The figure shows three views and two pictorial views of one solid part (mm, origin at its lowest corner). Answer the questions. A direction names the side the tool comes from. Give positions to 0.01 mm unless a question says otherwise; leave off trailing zeros. Write each loop counter-clockwise with the first axis right and the second up, starting at its lowest first coordinate (ties: lowest second). Pieces come first, ordered by that corner, then holes. Notation, with made-up numbers: (82.25, -27) -> (89.25, -27) arc R23 ccw to (89.25, 8) -> close; hole circle Ø10 at (-34, 67). An arc over 180 degrees is marked (long way). Write item = value, one per line. Start each with the question number.
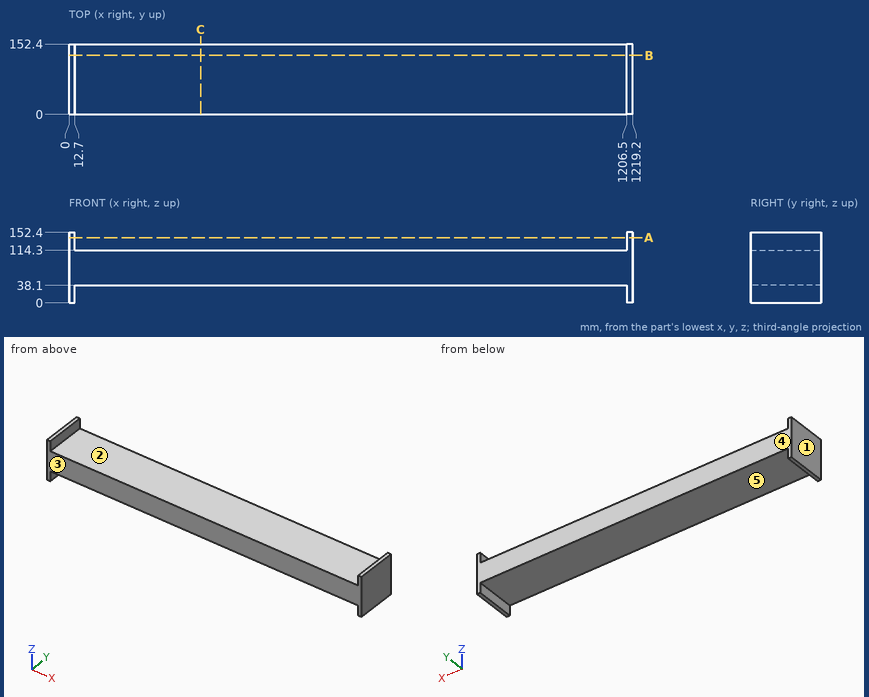
(1) For the marked faces 1 and 2, determine the directions among +Z, -Z, +X, -X, +Y, -Y from which every point of the face is accessible in a straight line to the end or side of a thin tool.
(2) This flat-tipped pin is pushed along its axis until it touches: pin 1 (4 mm diameter, centred on x = 228.5, y = 86, fed in from +Z). Where does it stop, or does it pass through?
(3) Find the intervals of material crossed by line 1 along X through (y, z) = (17.5, 134); line 2 along Z through (x, y) = (523.5, 63.5), in increasing order.
(4) A cutting plane is placed at C-C, the plane x = 285. Write down the section's boundary in (y, z).
(5) Determine the mould class of the marked faces 3, 4 and 5 for opening direction Y: pulls with the +Y half, pulls with the -Y half, needs draft (parallel to the pull), parting line crosses it, or undercut.
(6) A cutting plane is placed at B-B, the plane y = 128. Write down the section's boundary in (x, z), then the cut area to 3 significant figures.
(7) A cutting plane is placed at A-A, the plane z = 141. Write down the section's boundary in (x, y).
Results list:
q1.face_1 = +Z, -Z, -X, +Y, -Y
q1.face_2 = +Z, +Y, -Y
q2.pin_1 = 114.3
q3.line_1 = 0 to 12.7, 1206.5 to 1219.2
q3.line_2 = 38.1 to 114.3
q4.outline = (0, 38.1) -> (152.4, 38.1) -> (152.4, 114.3) -> (0, 114.3) -> close
q5.face_3 = pulls with the -Y half
q5.face_4 = pulls with the +Y half
q5.face_5 = needs draft
q6.outline = (0, 0) -> (12.7, 0) -> (12.7, 38.1) -> (1206.5, 38.1) -> (1206.5, 0) -> (1219.2, 0) -> (1219.2, 152.4) -> (1206.5, 152.4) -> (1206.5, 114.3) -> (12.7, 114.3) -> (12.7, 152.4) -> (0, 152.4) -> close
q6.area = 94,800 mm²
q7.outline = (0, 0) -> (12.7, 0) -> (12.7, 152.4) -> (0, 152.4) -> close; (1206.5, 0) -> (1219.2, 0) -> (1219.2, 152.4) -> (1206.5, 152.4) -> close
